from build123d import *

# Parameters (mm, degrees)
SKETCH1_R               = 7.5
BOSS_EXTRUDE1_DEPTH     = 55
CUT_EXTRUDE2_DEPTH      = 57.013391256
SKETCH4_R               = 7.5
SKETCH4_R_2             = 4
BOSS_EXTRUDE2_DEPTH     = 2
LPATTERN1_COUNT         = 2
LPATTERN1_PITCH         = 57
SKETCH6_R               = 3
SKETCH6_R_2             = 1.5
BOSS_EXTRUDE3_DEPTH     = 1.5
SKETCH7_W               = 27
SKETCH7_H               = 7.5
CUT_EXTRUDE3_DEPTH      = 60.055059055
CUT_EXTRUDE3_DEPTH_BACK = 60.055059055


with BuildPart() as part:
    # Sketch1 → Boss-Extrude1 (new body)
    with BuildSketch(Plane(origin=(0, 0, 0), x_dir=(1, 0, 0), z_dir=(0, 1, 0))):
        with Locations(Location((0, 0, 0), (0, 0, 270))):
            Circle(SKETCH1_R)
    extrude(amount=BOSS_EXTRUDE1_DEPTH)

    # Sketch3 → Cut-Extrude2 (cut, through all)
    with BuildSketch(Plane(origin=(0, 55, 0), x_dir=(1, 0, 0), z_dir=(0, 1, 0))):
        with BuildLine():
            Line((-0.407679482, 4.574145986), (-1, 5.408326913))
            ThreePointArc((-1, 5.408326913), (-2.104758878, 5.081337429), (-3.117157854, 4.531371416))
            Line((-3.117157854, 4.531371416), (-2.946136719, 3.522682571))
            ThreePointArc((-2.946136719, 3.522682571), (-3.085548023, 3.085548023), (-3.522682571, 2.946136719))
            Line((-3.522682571, 2.946136719), (-4.531371416, 3.117157854))
            ThreePointArc((-4.531371416, 3.117157854), (-5.081337429, 2.104758878), (-5.408326913, 1))
            Line((-5.408326913, 1), (-4.574145986, 0.407679482))
            ThreePointArc((-4.574145986, 0.407679482), (-4.363623861, 0), (-4.574145986, -0.407679482))
            Line((-4.574145986, -0.407679482), (-5.408326913, -1))
            ThreePointArc((-5.408326913, -1), (-5.081337429, -2.104758878), (-4.531371416, -3.117157854))
            Line((-4.531371416, -3.117157854), (-3.522682571, -2.946136719))
            ThreePointArc((-3.522682571, -2.946136719), (-3.085548023, -3.085548023), (-2.946136719, -3.522682571))
            Line((-2.946136719, -3.522682571), (-3.117157854, -4.531371416))
            ThreePointArc((-3.117157854, -4.531371416), (-2.104758878, -5.081337429), (-1, -5.408326913))
            Line((-1, -5.408326913), (-0.407679482, -4.574145986))
            ThreePointArc((-0.407679482, -4.574145986), (0, -4.363623861), (0.407679482, -4.574145986))
            Line((0.407679482, -4.574145986), (1, -5.408326913))
            ThreePointArc((1, -5.408326913), (2.104758878, -5.081337429), (3.117157854, -4.531371416))
            Line((3.117157854, -4.531371416), (2.946136719, -3.522682571))
            ThreePointArc((2.946136719, -3.522682571), (3.085548023, -3.085548023), (3.522682571, -2.946136719))
            Line((3.522682571, -2.946136719), (4.531371416, -3.117157854))
            ThreePointArc((4.531371416, -3.117157854), (5.081337429, -2.104758878), (5.408326913, -1))
            Line((5.408326913, -1), (4.574145986, -0.407679482))
            ThreePointArc((4.574145986, -0.407679482), (4.363623861, 0), (4.574145986, 0.407679482))
            Line((4.574145986, 0.407679482), (5.408326913, 1))
            ThreePointArc((5.408326913, 1), (5.081337429, 2.104758878), (4.531371416, 3.117157854))
            Line((4.531371416, 3.117157854), (3.522682571, 2.946136719))
            ThreePointArc((3.522682571, 2.946136719), (3.085548023, 3.085548023), (2.946136719, 3.522682571))
            Line((2.946136719, 3.522682571), (3.117157854, 4.531371416))
            ThreePointArc((3.117157854, 4.531371416), (2.104758878, 5.081337429), (1, 5.408326913))
            Line((1, 5.408326913), (0.407679482, 4.574145986))
            ThreePointArc((0.407679482, 4.574145986), (0, 4.363623861), (-0.407679482, 4.574145986))
        make_face()
    extrude(amount=-CUT_EXTRUDE2_DEPTH, mode=Mode.SUBTRACT)

    # Sketch4 → Boss-Extrude2 (add)
    with BuildSketch(Plane(origin=(0, 0, 0), x_dir=(1, 0, 0), z_dir=(0, 1, 0))):
        with Locations(Location((0, 0, 0), (0, 0, 270))):
            Circle(SKETCH4_R)
        with Locations(Location((0, 0, 0), (0, 0, 270))):
            Circle(SKETCH4_R_2, mode=Mode.SUBTRACT)
    boss_extrude2 = extrude(amount=-BOSS_EXTRUDE2_DEPTH)

    # LPattern1: Boss-Extrude2 ×2
    with Locations(*[(0, i * LPATTERN1_PITCH, 0) for i in range(1, LPATTERN1_COUNT)]):
        add(boss_extrude2)

    # Sketch6 → Boss-Extrude3 (add, symmetric)
    with BuildSketch(Plane.XY):
        with BuildLine():
            Line((-6, 24.5), (-6, 30.5))
            Line((-6, 30.5), (-10.5, 30.5))
            ThreePointArc((-10.5, 30.5), (-8.378679656, 29.621320344), (-7.5, 27.5))
            ThreePointArc((-7.5, 27.5), (-8.378679656, 25.378679656), (-10.5, 24.5))
            Line((-10.5, 24.5), (-6, 24.5))
        make_face()
        with BuildLine():
            Line((10.5, 30.5), (6, 30.5))
            Line((6, 30.5), (6, 24.5))
            Line((6, 24.5), (10.499999991, 24.5))
            ThreePointArc((10.499999991, 24.5), (7.5, 27.500000005), (10.5, 30.5))
        make_face()
        with Locations((10.5, 27.5)):
            Circle(SKETCH6_R)
        with Locations((10.5, 27.5)):
            Circle(SKETCH6_R_2, mode=Mode.SUBTRACT)
        with Locations((-10.5, 27.5)):
            Circle(SKETCH6_R)
        with Locations((-10.5, 27.5)):
            Circle(SKETCH6_R_2, mode=Mode.SUBTRACT)
    extrude(amount=BOSS_EXTRUDE3_DEPTH, both=True)

    # Sketch7 → Cut-Extrude3 (cut, two sides)
    with BuildSketch(Plane(origin=(0, 0, 0), x_dir=(1, 0, 0), z_dir=(0, 1, 0))) as cut_extrude3_sk:
        with Locations((0, -3.75)):
            Rectangle(SKETCH7_W, SKETCH7_H)
    extrude(amount=CUT_EXTRUDE3_DEPTH, mode=Mode.SUBTRACT)
    extrude(cut_extrude3_sk.sketch, amount=-CUT_EXTRUDE3_DEPTH_BACK, mode=Mode.SUBTRACT)


solid = part.part
Could you check a few things on this model? Use its own coordinates, in mm. A direction names the side the tool comes from. Give positions to 0.01 mm unless a question says otherwise; leave off trailing zeros. Loops run counter-clockwise (first coordinate to the right, second up) from the corner with the lowest first, then second, coordinate; pieces in that order, holes last. Notation, with made-up numbers: (84, 79) -> (132, 79) arc R27 cw to (132, 100) -> close; hole circle Ø7 at (-33.5, -10). An arc over 180 degrees is marked (long way). Answer as CSV lines item,"result". Start each with the question number.
(1) If we section it at A-A on y = 27.5: Count the separate pieces of the cut face and the enclosed holes in it, then the cut area to 3 significant figures.
(2) We'd pull the mould along Y, two halves only. Please class faces 4 (the flat face through (-9, 26, -1.5)), 5 (the flat face through (-0.8, 55, -4.1)), 6 (the flat face through (-9, 30.5, -1)): released by +Y, released by -Y, zero draft, split by the parting line, or undercut.
(3) If we section it at C-C on x = 6.5: Write out the boundary of the cut face in (y, z).
(4) I need wall thicknesses on probe 1 along Y at (x, z) = (10.5, -0.45); probe 2 along X at (y, z) = (27.5, -0.8); probe 3 along X at (y, z) = (27.5, -0.55). Which ranges of each line are inside material? Lowest first, please.
(5) Which directions (+Z, -Z, +X, -X, +Y, -Y) give clear straight access to the entire face, cutting with the end or side of a thin tool? Please do faces 1 (the flat face through (-3.033, 27.885, -4.034)), 2 (the flat face through (9, 28.2, -1.5)), 3 (the flat face through (-7, 27, 0)).
(6) I'm going to push flat-ended pins straight in: pin 1 Ø4.5 at (x, z) = (-1.5, -3.5) entering from +Y; pin 2 Ø3 at (y, z) = (35.5, -2) entering from -X; pin 3 Ø1.2 at (x, z) = (-8.5, -0.5) entering from -Y; pin 4 Ø1.8 at (x, y) = (-11.5, 27) entering from -Z. Where does each tip first touch, or does it pass through?
(7) If we section it at B-B on y = 52: Write out the boundary of the cut face in (x, z), then the cut area to 3 significant figures.
Computed:
1,separate pieces,"3"
1,enclosed holes,"0"
1,area,"55.7 mm2"
2,face 4,"zero draft"
2,face 5,"undercut"
2,face 6,"released by +Y"
3,outline,"(-2, -3.74) -> (57, -3.74) -> (57, 0) -> (-2, 0) -> close"
4,probe 1,"y = 24.5 to 26, 29 to 30.5"
4,probe 2,"x = -13.5 to -12, -9 to -5.13, 5.13 to 9, 12 to 13.5"
4,probe 3,"x = -13.5 to -12, -9 to -4.77, 4.77 to 9, 12 to 13.5"
5,face 1,"none"
5,face 2,"-Z, +X, +Y, -Y"
5,face 3,"+Z, +X, -X, +Y, -Y"
6,pin 1,"stops at y = 57"
6,pin 2,"stops at x = -7.48"
6,pin 3,"stops at y = 24.5"
6,pin 4,"stops at z = -1.5"
7,outline,"(-7.5, 0) arc R7.5 ccw to (7.5, 0) -> (4.36, 0) arc R0.5 ccw to (4.57, -0.41) -> (5.41, -1) arc R5.5 cw to (4.53, -3.12) -> (3.52, -2.95) arc R0.5 ccw to (2.95, -3.52) -> (3.12, -4.53) arc R5.5 cw to (1, -5.41) -> (0.41, -4.57) arc R0.5 ccw to (-0.41, -4.57) -> (-1, -5.41) arc R5.5 cw to (-3.12, -4.53) -> (-2.95, -3.52) arc R0.5 ccw to (-3.52, -2.95) -> (-4.53, -3.12) arc R5.5 cw to (-5.41, -1) -> (-4.57, -0.41) arc R0.5 ccw to (-4.36, 0) -> close"
7,area,"46.5 mm2"
